Autodesk Inventor part; units mm, degrees
ref_plane "YZ Plane" through (0, 0, 0) normal (1, 0, 0) x (0, 1, 0)
ref_plane "XZ Plane" through (0, 0, 0) normal (0, 1, 0) x (-1, 0, 0)
ref_plane "XY Plane" through (0, 0, 0) normal (0, 0, 1) x (1, 0, 0)
ref_plane "Arbeitsebene1" through (0, 0, 0) normal (0, 0, 1) x (1, 0, 0)
sketch "Skizze1" plane through (0, 0, 0) normal (0, 0, 1) x (1, 0, 0)
  spline S0 degree 3 poles (34.5, 0) (34.4922, -0.0784) (34.4879, -0.2047) (34.5533, -0.4702) (34.6001, -0.5784) (34.7323, -0.7826) (34.8194, -0.8753) (34.994, -1.0048) (35.1117, -1.0785) (35.3805, -1.1607) (35.4924, -1.1779) (35.724, -1.1797) (35.8424, -1.1625) (35.9562, -1.1277) knots -0.341572 -0.341572 -0.341572 -0.341572 -0.254859 -0.254859 -0.189973 -0.189973 -0.120019 -0.120019 -0.069482 -0.069482 -0.03569 -0.03569 0 0 0 0 construction
  circle A0 centre (35.5, 0) radius 1 construction
  circle A1 centre (-35.5, 0) radius 1 construction
  line L0 (-36.5594, -4.5) -> (36.5594, -4.5) construction
  line L1 (37.5, -3.5594) -> (37.5, 3.5594) construction
  line L2 (-36.5594, 4.5) -> (36.5594, 4.5) construction
  line L3 (-37.5, -3.5594) -> (-37.5, 3.5594) construction
  line L4 (-36.95, 3.5319) -> (-36.95, -3.5319) construction
  arc A2 (-36.5319, -3.95) -> (-36.95, -3.5319) centre (-37.1503, -4.1503) ccw construction
  line L5 (-36.5319, -3.95) -> (36.5319, -3.95) construction
  arc A3 (36.95, -3.5319) -> (36.5319, -3.95) centre (37.1503, -4.1503) ccw construction
  line L6 (36.95, 3.5319) -> (36.95, -3.5319) construction
  arc A4 (36.5319, 3.95) -> (36.95, 3.5319) centre (37.1503, 4.1503) ccw construction
  line L7 (-36.5319, 3.95) -> (36.5319, 3.95) construction
  arc A5 (-36.95, 3.5319) -> (-36.5319, 3.95) centre (-37.1503, 4.1503) ccw construction
  spline S1 degree 3 poles (-36.5, 0) (-36.5078, -0.0784) (-36.5121, -0.2047) (-36.4467, -0.4702) (-36.3999, -0.5784) (-36.2677, -0.7826) (-36.1806, -0.8753) (-36.006, -1.0048) (-35.8883, -1.0785) (-35.6195, -1.1607) (-35.5076, -1.1779) (-35.276, -1.1797) (-35.1576, -1.1625) (-35.0438, -1.1277) knots -0.341572 -0.341572 -0.341572 -0.341572 -0.254859 -0.254859 -0.189973 -0.189973 -0.120019 -0.120019 -0.069482 -0.069482 -0.03569 -0.03569 0 0 0 0 construction
  arc A6 (-35.5, 1) -> (-36.5, 0) centre (-35.5, 0) ccw construction
  spline S2 degree 3 poles (-34.3787, -0.4718) (-34.3466, -0.3696) (-34.3281, -0.2637) (-34.32, -0.0752) (-34.3224, 0.0413) (-34.3918, 0.3184) (-34.4553, 0.4524) (-34.6302, 0.687) (-34.7395, 0.7855) (-34.9556, 0.9143) (-35.0636, 0.9616) (-35.2916, 1.0075) (-35.3964, 1.012) (-35.5, 1) knots -0.292776 -0.292776 -0.292776 -0.292776 -0.226562 -0.226562 -0.176122 -0.176122 -0.122734 -0.122734 -0.069758 -0.069758 -0.031291 -0.031291 0 0 0 0 construction
  arc A7 (-35.0438, -1.1277) -> (-34.3787, -0.4718) centre (-35.5, 0) ccw construction
  spline S3 degree 3 poles (34.5, 0) (34.4922, -0.0784) (34.4879, -0.2047) (34.5533, -0.4702) (34.6001, -0.5784) (34.7323, -0.7826) (34.8194, -0.8753) (34.994, -1.0048) (35.1117, -1.0785) (35.3805, -1.1607) (35.4924, -1.1779) (35.724, -1.1797) (35.8424, -1.1625) (35.9562, -1.1277) knots -0.341572 -0.341572 -0.341572 -0.341572 -0.254859 -0.254859 -0.189973 -0.189973 -0.120019 -0.120019 -0.069482 -0.069482 -0.03569 -0.03569 0 0 0 0 construction
  arc A8 (35.5, 1) -> (34.5, 0) centre (35.5, 0) ccw construction
  spline S4 degree 3 poles (36.6213, -0.4718) (36.6534, -0.3696) (36.6719, -0.2637) (36.68, -0.0752) (36.6776, 0.0413) (36.6082, 0.3184) (36.5447, 0.4524) (36.3698, 0.687) (36.2605, 0.7855) (36.0444, 0.9143) (35.9364, 0.9616) (35.7084, 1.0075) (35.6036, 1.012) (35.5, 1) knots -0.292776 -0.292776 -0.292776 -0.292776 -0.226562 -0.226562 -0.176122 -0.176122 -0.122734 -0.122734 -0.069758 -0.069758 -0.031291 -0.031291 0 0 0 0 construction
  arc A9 (35.9562, -1.1277) -> (36.6213, -0.4718) centre (35.5, 0) ccw construction
  line L8 (-33.5, 1) -> (-33.5, -1) construction
  arc A10 (-33, 1.5) -> (-33.5, 1) centre (-33, 1) ccw construction
  line L9 (33, 1.5) -> (-33, 1.5) construction
  arc A11 (33.5, 1) -> (33, 1.5) centre (33, 1) ccw construction
  line L10 (33.5, -1) -> (33.5, 1) construction
  arc A12 (33, -1.5) -> (33.5, -1) centre (33, -1) ccw construction
  line L11 (-33, -1.5) -> (33, -1.5) construction
  arc A13 (-33.5, -1) -> (-33, -1.5) centre (-33, -1) ccw construction
  line L12 (40.5, -6.5) -> (-40.5, -6.5)
  line L13 (-40.5, -6.5) -> (-40.5, 27)
  line L14 (-40.5, 27) -> (40.5, 27)
  line L15 (40.5, 27) -> (40.5, -6.5)
  circle A14 centre (35.5, 0) radius 1.25
  circle A15 centre (-35.5, 0) radius 1.25
  arc A16 (33, -2) -> (34, -1) centre (33, -1) ccw
  line L16 (34, -1) -> (34, 1)
  arc A17 (34, 1) -> (33, 2) centre (33, 1) ccw
  line L17 (33, 2) -> (-33, 2)
  arc A18 (-33, 2) -> (-34, 1) centre (-33, 1) ccw
  line L18 (-34, 1) -> (-34, -1)
  arc A19 (-34, -1) -> (-33, -2) centre (-33, -1) ccw
  line L19 (-33, -2) -> (33, -2)
  point P0 (0, 0)
  dimension "d0" = 5
  dimension "d1" = 5
  dimension "d2" = 2
  dimension "d3" = 27
  dimension "d4" = 2.5
  dimension "d5" = 2.5
extrude "Extrusion1" add sketch "Skizze1" along normal blind 2
fillet "Rundung1" radius 5 2 edges at (40.5, -6.5, 1) (-40.5, -6.5, 1)
sketch "Skizze2" plane through (0, 0, 0) normal (0, 0, -1) x (-1, 0, 0)
  line L0 (-40.5, 27) -> (40.5, 27) construction
  line L1 (40.5, 27) -> (40.5, -1.5) construction
  line L2 (-40.5, -1.5) -> (-40.5, 27) construction
  line L3 (40.5, 27) -> (-40.5, 27)
  line L4 (-40.5, 27) -> (-40.5, 25)
  line L5 (-40.5, 25) -> (40.5, 25)
  line L6 (40.5, 25) -> (40.5, 27)
  point P0 (0, 0)
  dimension "d9" = 2
extrude "Extrusion2" add sketch "Skizze2" along normal blind 20
sketch "Skizze3" plane through (40.5, -1.5, 2) normal (1, 0, 0) x (0, 0, -1)
  line L0 (2, 0) -> (0, 0) construction
  line L1 (2, 0) -> (2, 26.5)
  line L2 (2, 26.5) -> (22, 26.5)
  line L3 (22, 28.5) -> (22, 26.5) construction
  line L4 (0, 28.5) -> (22, 28.5) construction
  line L5 (0, 0) -> (0, 28.5) construction
  line L6 (2, 0) -> (22, 26.5)
  point P0 (2, 1.5)
extrude "Extrusion3" add sketch "Skizze3" against normal blind 1
sketch "Skizze4" plane through (-40.5, -1.5, 2) normal (-1, 0, 0) x (0, 0, 1)
  line L0 (-22, 26.5) -> (-2, 26.5)
  line L1 (-22, 26.5) -> (-2, 0)
  line L2 (-2, 26.5) -> (-2, 0)
  point P0 (-2, 1.5)
extrude "Extrusion4" add sketch "Skizze4" against normal blind 1
sketch "Skizze5" plane through (39.5, 25, -20) normal (0, -1, 0) x (1, 0, 0)
  line L0 (-0.5716, 5) -> (-194.7619, 5) construction
  line L1 (-7.5, 5) -> (-22.5, 5) construction
  line L2 (-7.5, 6.75) -> (-22.5, 6.75)
  line L3 (-22.5, 3.25) -> (-7.5, 3.25)
  arc A0 (-7.5, 3.25) -> (-7.5, 6.75) centre (-7.5, 5) ccw
  arc A1 (-22.5, 6.75) -> (-22.5, 3.25) centre (-22.5, 5) ccw
  line L4 (-56.5, 5) -> (-71.5, 5) construction
  line L5 (-56.5, 6.75) -> (-71.5, 6.75)
  line L6 (-71.5, 3.25) -> (-56.5, 3.25)
  arc A2 (-56.5, 3.25) -> (-56.5, 6.75) centre (-56.5, 5) ccw
  arc A3 (-71.5, 6.75) -> (-71.5, 3.25) centre (-71.5, 5) ccw
  line L7 (0, 0) -> (-79, 0)
  line L8 (0, 0) -> (0, 20)
  line L9 (-79, 20) -> (-79, 0)
  point P0 (-39.5, 20)
  point P1 (-15, 5)
  point P2 (-64, 5)
  dimension "d16" = 3.5
  dimension "d17" = 15
  dimension "d18" = 5
  dimension "d19" = 15
  dimension "d20" = 15
extrude "Extrusion5" cut sketch "Skizze5" against normal through all
properties part number "Halterung_Winkel"
For this review, take the finished solid that the model builds, in its own axes (mm). A direction names the side the tool comes from. Round coordinates to 2 decimals unless told otherwise and drop trailing zeros. Loops run counter-clockwise (first coordinate to the right, second up) from the corner with the lowest first, then second, coordinate; pieces in that order, holes last. Notation, with made-up numbers: (32.5, 32) - (57.5, 32) arc R22 ccw to (57.5, 54) - close; hole circle Ø5 at (2.25, 73.5). An arc over 180 degrees is marked (long way). Use one line per item in the form item = value.
1) Tool access review of faces 1 (the face through (-24, 26, -13.25)), 2 (the face through (-1, 10, 2)), 3 (the face through (34, 0, 1)), 4 (the face through (0, -6.5, 1)), 5 (the face through (1, 25, -10)): name each direction out of +Z, -Z, +X, -X, +Y, -Y from which nothing blocks a thin tool from reaching the whole face with its end or side.
Solutions:
face_1 = +Y, -Y
face_2 = +Z, +X, -X, +Y, -Y
face_3 = +Z, -Z
face_4 = +Z, -Z, +X, -X, -Y
face_5 = -Z, -Y
2) We need section B-B on x = -11. Write out the cut boundary in (y, z).
Solutions:
outline = (-6.5, 0) - (-2, 0) - (-2, 2) - (-6.5, 2) - close; (2, 0) - (25, 0) - (25, -20) - (27, -20) - (27, 2) - (2, 2) - close
3) Wall thickness on probe 1 along X at (y, z) = (9.5, -4.75); probe 2 along Y at (x, z) = (35.5, 0.65); probe 3 along Z at (x, y) = (22, 25.5): over which ranges is each line inside the solid? List them lowest first.
Solutions:
probe_1 = -40.5 to -39.5, 39.5 to 40.5
probe_2 = -6.5 to -1.25, 1.25 to 27
probe_3 = -20 to -16.75, -13.25 to 2
4) We need section D-D on y = 0. Write out the cut boundary in (x, z), then the cut area to 3 significant figures.
Solutions:
outline = (-40.5, -1.13) - (-39.5, -1.13) - (-39.5, 0) - (-36.75, 0) - (-36.75, 2) - (-40.5, 2) - close; (-34.25, 0) - (-34, 0) - (-34, 2) - (-34.25, 2) - close; (34, 0) - (34.25, 0) - (34.25, 2) - (34, 2) - close; (36.75, 0) - (39.5, 0) - (39.5, -1.13) - (40.5, -1.13) - (40.5, 2) - (36.75, 2) - close
area = 18.3 mm2
5) Mouldability with a two-part tool opening along Z and no side actions: class faces 6 (the face through (24, 26, -16.75)), 7 (the face through (1, 26, -20)), 8 (the face through (39.5, 15, -8)), 9 (the face through (33.75, 25.99, -15.04)) as pulls with the +Z half, pulls with the -Z half, needs draft (parallel to the pull), parting line crosses it, or undercut.
Solutions:
face_6 = undercut
face_7 = pulls with the -Z half
face_8 = needs draft
face_9 = undercut
6) Clearance check with flat-ended pins moving along their axes: P1, Ø10, axis at x = -16, y = 13, coming from the -Z side; P2, Ø6, axis at x = -6, y = -1.5, coming from the +Z side; P3, Ø1, axis at x = 22, z = -5, coming from the -Y side. State where each tip first meets the part, or that it passes through.
Solutions:
P1 = 0
P2 = 2
P3 = 25
7) We need section A-A on x = 21. Write out the cut boundary in (y, z), then the cut area to 3 significant figures.
Solutions:
outline = (-6.5, 0) - (-2, 0) - (-2, 2) - (-6.5, 2) - close; (2, 0) - (25, 0) - (25, -13.25) - (27, -13.25) - (27, 2) - (2, 2) - close; (25, -20) - (27, -20) - (27, -16.75) - (25, -16.75) - close
area = 92.0 mm2
8) We need section C-C on z = -15. Write out the cut boundary in (x, y) (3 decimals), then the cut area to 3 significant figures.
Solutions:
outline = (-40.5, 18.375) - (-39.5, 18.375) - (-39.5, 25) - (-33.75, 25) - (-33.75, 27) - (-40.5, 27) - close; (-15.25, 25) - (15.25, 25) - (15.25, 27) - (-15.25, 27) - close; (33.75, 25) - (39.5, 25) - (39.5, 18.375) - (40.5, 18.375) - (40.5, 27) - (33.75, 27) - close
area = 101 mm2
